Verification items for the finished model (mm, model axes). Face numbers are marked on the shaded views. A direction names the side the tool comes from. Coordinates: 2 decimals unless noted, no trailing zeros. Order: outer loops, then holes, each group sorted by start corner. A loop starts at its lowest first (then second) coordinate and runs counter-clockwise, first axis right, second up. Notation, with made-up numbers: M -29.75,-23.75 L -8.75,-23.75 A27 cw -8.75,-5.75 Z; hole C 32,87.5 d4. An arc over 180 degrees is marked long. Return JSON: item names as keys, results as strings. Group by question number.
1. Section check B-B, the plane y = 38.5. Record the cut outline in (x, z).
2. Section check C-C, the plane x = -17. Record the cut outline in (y, z), plus the area to 3 significant figures.
3. Material ranges on line 1 along Z through (x, y) = (-7.5, 3.5); line 2 along Z through (x, y) = (-3, 3.5); line 3 along Z through (x, y) = (0, 1), recorded low to high.
4. Gauge pin test, flat ends, axial feed: pin 1 (5.5 mm diameter, centred on x = -2, z = -1, fed in from +Y); pin 2 (3 mm diameter, centred on x = 13, z = -14.5, fed in from -Y); pin 3 (3 mm diameter, centred on x = -22, y = 18.5, fed in from -Z); pin 4 (7 mm diameter, centred on x = -16.59, y = 10, fed in from +Z). Record the tip position at first contact, or that the pin passes through.
5. Set-up check for the marked faces 1, 2 and 3: record each of +Z, -Z, +X, -X, +Y, -Y from which the full face is reachable in a straight line by a thin tool's end or side.
6. Mould release check, pull along Z, two halves, no side actions. Record for the marked faces 4, 5 and 6: +Z half, -Z half, draft (parallel to the pull), parting line (faces both ways), or undercut.
7. Section check A-A, the plane y = 8. Record the cut outline in (x, z), plus the area to 3 significant figures.
8. Section check D-D, the plane y = 16.5. Record the cut outline in (x, z).
```python
from build123d import *

# Parameters (mm, degrees)
SKETCH_1_R          = 2.15
EXTRUDE_1_DEPTH     = 6
EXTRUDE_2_DEPTH     = 35
SKETCH_3_W          = 63
SKETCH_3_H          = 21
CUT_EXTRUDE_1_DEPTH = 21
SKETCH_4_R          = 2.75
CUT_EXTRUDE_2_DEPTH = 87.609201921
CHAMFER_1_SIZE      = 9.5
CHAMFER_1_SIZE_2    = 9.174043361
CUT_EXTRUDE_START   = -10
SKETCH_5_R          = 4.25
CUT_EXTRUDE_3_DEPTH = 5
SKETCH_6_R          = 2.75
CUT_EXTRUDE_4_DEPTH = 78.360370477
CUT_EXTRUDE_START_2 = -4
SKETCH_7_R          = 4.25
CUT_EXTRUDE_5_DEPTH = 5
SKETCH_8_R          = 2.75
CUT_EXTRUDE_6_DEPTH = 64.20427816
SKETCH_10_R         = 4.25
CUT_EXTRUDE_7_DEPTH = 15.5
SKETCH_11_R         = 4.25
CUT_EXTRUDE_8_DEPTH = 20
CUT_EXTRUDE_9_DEPTH = 3


with BuildPart() as part:
    # Эскиз1 → Бобышка-Вытянуть1 (new body)
    with BuildSketch(Plane(origin=(0, 0, 0), x_dir=(1, 0, 0), z_dir=(0, 1, 0))):
        Polygon((-31.737099952, -43.025037564), (41.262900048, -43.025037564), (41.262900048, -20.025037564), (11.262900048, -13.109402144), (11.262900048, 28.974962436), (-31.737099952, 28.974962436), align=None)
        with Locations(Location((-10.237099952, 19.879797383, 0), (0, 0, 270))):
            Circle(SKETCH_1_R, mode=Mode.SUBTRACT)
        with Locations(Location((0, 0, 0), (0, 0, 270))):
            Circle(SKETCH_1_R, mode=Mode.SUBTRACT)
    extrude(amount=EXTRUDE_1_DEPTH)

    # Эскиз2 → Бобышка-Вытянуть2 (add)
    with BuildSketch(Plane(origin=(0, 6, 0), x_dir=(1, 0, 0), z_dir=(0, 1, 0))):
        Polygon((41.262900048, -20.025037564), (11.262900048, -13.109402144), (-31.737099952, -13.109402144), (-31.737099952, -43.025037564), (41.262900048, -43.025037564), align=None)
    extrude(amount=EXTRUDE_2_DEPTH)

    # Эскиз3 → Вырез-Вытянуть1 (cut)
    with BuildSketch(Plane(origin=(0, 41, 0), x_dir=(1, 0, 0), z_dir=(0, 1, 0))):
        with Locations((9.762900048, -32.525037564)):
            Rectangle(SKETCH_3_W, SKETCH_3_H)
    extrude(amount=-CUT_EXTRUDE_1_DEPTH, mode=Mode.SUBTRACT)

    # Эскиз4 → Вырез-Вытянуть2 (cut, through all)
    with BuildSketch(Plane(origin=(-21.737099952, 0, 0), x_dir=(0, 0, -1), z_dir=(1, 0, 0))):
        with Locations((-32.525037564, 30.5)):
            Circle(SKETCH_4_R)
    extrude(amount=-CUT_EXTRUDE_2_DEPTH, mode=Mode.SUBTRACT)

    # Фаска1
    # the kernel refuses this chamfer: 9.5, 9.174043361 mm, written as the material it takes off along each edge
    with BuildSketch(Plane(origin=(-31.737099952, 41, -11.332881065), x_dir=(-0.026999337430198715, -0.9996354514413394, 0), z_dir=(0, 0, 1))) as chamfer_1_piece_1:
        Polygon((CHAMFER_1_SIZE * 0.999635451441, CHAMFER_1_SIZE * 0.0269993374302), (-CHAMFER_1_SIZE_2 * 0.0269993374292, CHAMFER_1_SIZE_2 * 0.999635451405), (0, 0), align=None)
    extrude(amount=78.800201839, mode=Mode.SUBTRACT)

    # Эскиз5 → Вырез-Вытянуть3 (cut)
    with BuildSketch(Plane(origin=(-21.737099952, 0, 0), x_dir=(0, 0, -1), z_dir=(1, 0, 0)).offset(CUT_EXTRUDE_START)):
        with Locations(Location((-32.525037564, 30.5, 0), (0, 0, 166.391039369))):
            Circle(SKETCH_5_R)
    extrude(amount=CUT_EXTRUDE_3_DEPTH, mode=Mode.SUBTRACT)

    # Эскиз6 → Вырез-Вытянуть4 (cut, through all)
    with BuildSketch(Plane.XY.offset(22.025037564)):
        with Locations((-9.495708976, 30.5)):
            Circle(SKETCH_6_R)
        with Locations((22.785725254, 30.5)):
            Circle(SKETCH_6_R)
    extrude(amount=-CUT_EXTRUDE_4_DEPTH, mode=Mode.SUBTRACT)

    # Эскиз7 → Вырез-Вытянуть5 (cut)
    with BuildSketch(Plane.XY.offset(22.025037564).offset(CUT_EXTRUDE_START_2)):
        with Locations((-9.495708976, 30.5)):
            Circle(SKETCH_7_R)
        with Locations((22.785725254, 30.5)):
            Circle(SKETCH_7_R)
    extrude(amount=-CUT_EXTRUDE_5_DEPTH, mode=Mode.SUBTRACT)

    # Эскиз8 → Вырез-Вытянуть6 (cut, through all)
    with BuildSketch(Plane(origin=(0, 20, 0), x_dir=(1, 0, 0), z_dir=(0, 1, 0))):
        with Locations(Location((-4.483206982, -32.525037564, 0), (0, 0, 270))):
            Circle(SKETCH_8_R)
        with Locations(Location((23.126402015, -32.525037564, 0), (0, 0, 270))):
            Circle(SKETCH_8_R)
    extrude(amount=-CUT_EXTRUDE_6_DEPTH, mode=Mode.SUBTRACT)

    # Эскиз10 → Вырез-Вытянуть7 (cut)
    with BuildSketch(Plane.XZ):
        with Locations(Location((23.126402015, 32.525037564, 0), (0, 0, 270))):
            Circle(SKETCH_10_R)
        with Locations(Location((-4.483206982, 32.525037564, 0), (0, 0, 270))):
            Circle(SKETCH_10_R)
    extrude(amount=-CUT_EXTRUDE_7_DEPTH, mode=Mode.SUBTRACT)

    # Эскиз11 → Вырез-Вытянуть8 (cut)
    with BuildSketch(Plane.XY.offset(43.025037564)):
        with Locations((-16.587099952, 10)):
            Circle(SKETCH_11_R)
    extrude(amount=-CUT_EXTRUDE_8_DEPTH, mode=Mode.SUBTRACT)

    # Эскиз12 → Вырез-Вытянуть9 (cut)
    with BuildSketch(Plane(origin=(0, 6, 0), x_dir=(1, 0, 0), z_dir=(0, 1, 0))):
        Polygon((-6.195648068, 19.879797383), (-8.21637401, 23.379797383), (-12.257825894, 23.379797383), (-14.278551837, 19.879797383), (-12.257825894, 16.379797383), (-8.21637401, 16.379797383), align=None)
        Polygon((4.041451884, 0), (2.020725942, 3.5), (-2.020725942, 3.5), (-4.041451884, 0), (-2.020725942, -3.5), (2.020725942, -3.5), align=None)
    extrude(amount=-CUT_EXTRUDE_9_DEPTH, mode=Mode.SUBTRACT)


solid = part.part
```
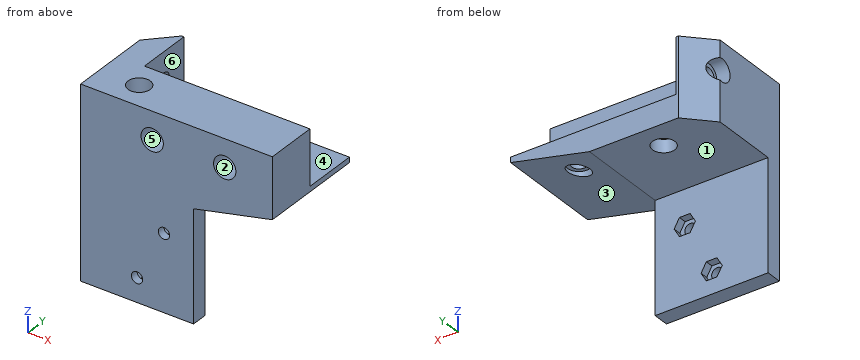
Answers follow:
{
 "1": {"outline": "M -24.98,13.11 L 11.26,13.11 L 41.26,20.03 L 41.26,22.03 L -21.74,22.03 L -21.74,43.03 L -24.98,43.03 Z"},
 "2": {"outline": "M 0,-28.97 L 6,-28.97 L 6,13.11 L 41,13.11 L 41,22.03 L 20,22.03 L 20,43.03 L 14.23,43.03 L 14.23,23.03 L 5.77,23.03 L 5.77,43.03 L 0,43.03 Z", "area": "869 mm^2"},
 "3": {"line 1": "-28.97 to -22.14, -17.62 to 29.53, 35.52 to 43.03", "line 2": "-28.97 to -1.8, 1.8 to 28.54, 36.51 to 43.03", "line 3": "-28.97 to -2.15, 2.15 to 43.03"},
 "4": {"pin 1": "y = 6", "pin 2": "through", "pin 3": "z = 13.11", "pin 4": "z = 23.03"},
 "5": {"face 1": "-Z, +X, -X, +Y", "face 2": "-Y", "face 3": "-Z, +X, +Y, -Y"},
 "6": {"face 4": "+Z half", "face 5": "undercut", "face 6": "draft"},
 "7": {"outline": "M -31.74,13.11 L 11.26,13.11 L 41.26,20.03 L 41.26,43.03 L -12.84,43.03 L -12.84,23.03 L -20.34,23.03 L -20.34,43.03 L -31.74,43.03 Z; hole C -4.48,32.53 d8.5; hole C 23.13,32.53 d8.5", "area": "1,820 mm^2"},
 "8": {"outline": "M -31.74,13.11 L 11.26,13.11 L 41.26,20.03 L 41.26,43.03 L -31.74,43.03 Z; hole C -4.48,32.53 d5.5; hole C 23.13,32.53 d5.5"}
}
